```python
from build123d import *

# Parameters (mm, degrees)
SKETCH1_R               = 1.350662837
BOSS_EXTRUDE1_DEPTH     = 3
BOSS_EXTRUDE2_OUTLINE_R = 1.350662837
BOSS_EXTRUDE2_DEPTH     = 5
BOSS_EXTRUDE2_START     = -18.821590418
BOSS_EXTRUDE2_2_DEPTH   = 37.643180836
FILLET1_R               = 0.5
SKETCH5_R               = 2.5
CUT_EXTRUDE1_DEPTH      = 25.78411334
FILLET2_R               = 0.5
FILLET3_R               = 1


with BuildPart() as part:
    # Sketch1 → Boss-Extrude1 (new body)
    with BuildSketch(Plane.XY):
        with BuildLine():
            Line((7.5, 18.821590418), (9.5, 18.821590418))
            Line((9.5, 18.821590418), (9.5, 17.821590418))
            Line((9.5, 17.821590418), (7.5, 15.821590418))
            Line((7.5, 15.821590418), (7.5, 11.821590418))
            ThreePointArc((7.5, 11.821590418), (14, 0), (7.5, -11.821590418))
            Line((7.5, -11.821590418), (7.5, -15.821590418))
            Line((7.5, -15.821590418), (9.5, -17.821590418))
            Line((9.5, -17.821590418), (9.5, -18.821590418))
            Line((9.5, -18.821590418), (7.5, -18.821590418))
            Line((7.5, -18.821590418), (-7.5, -18.821590418))
            Line((-7.5, -18.821590418), (-9.5, -18.821590418))
            Line((-9.5, -18.821590418), (-9.5, -17.821590418))
            Line((-9.5, -17.821590418), (-7.5, -15.821590418))
            Line((-7.5, -15.821590418), (-7.5, -11.821590418))
            ThreePointArc((-7.5, -11.821590418), (-14, 0), (-7.5, 11.821590418))
            Line((-7.5, 11.821590418), (-7.5, 15.821590418))
            Line((-7.5, 15.821590418), (-9.5, 17.821590418))
            Line((-9.5, 17.821590418), (-9.5, 18.821590418))
            Line((-9.5, 18.821590418), (-7.5, 18.821590418))
            Line((-7.5, 18.821590418), (7.5, 18.821590418))
        make_face()
        with Locations((-5, -8.660254038)):
            Circle(SKETCH1_R, mode=Mode.SUBTRACT)
        with Locations((10, 0)):
            Circle(SKETCH1_R, mode=Mode.SUBTRACT)
        with Locations((-5, 8.660254038)):
            Circle(SKETCH1_R, mode=Mode.SUBTRACT)
    extrude(amount=BOSS_EXTRUDE1_DEPTH)

    # Boss-Extrude2: read off the stored shape, not the designer's step
    # Boss-Extrude2 outline → Boss-Extrude2 (add)
    with BuildSketch(Plane(origin=(0, 0, 0), x_dir=(-1, 0, 0), z_dir=(0, 0, -1))):
        with BuildLine():
            Line((-7.5, 15.821590418), (-7.5, 11.821590418))
            ThreePointArc((-7.5, 11.821590418), (-14, 0), (-7.5, -11.821590418))
            Line((-7.5, -11.821590418), (-7.5, -15.821590418))
            Line((-7.5, -15.821590418), (-9.5, -17.821590418))
            Line((-9.5, -17.821590418), (-9.5, -18.821590418))
            Line((-9.5, -18.821590418), (9.5, -18.821590418))
            Line((9.5, -18.821590418), (9.5, -17.821590418))
            Line((9.5, -17.821590418), (7.5, -15.821590418))
            Line((7.5, -15.821590418), (7.5, -11.821590418))
            ThreePointArc((7.5, -11.821590418), (14, 0), (7.5, 11.821590418))
            Line((7.5, 11.821590418), (7.5, 15.821590418))
            Line((7.5, 15.821590418), (9.5, 17.821590418))
            Line((9.5, 17.821590418), (9.5, 18.821590418))
            Line((9.5, 18.821590418), (-9.5, 18.821590418))
            Line((-9.5, 18.821590418), (-9.5, 17.821590418))
            Line((-9.5, 17.821590418), (-7.5, 15.821590418))
        make_face()
        with Locations((5, -8.660254038)):
            Circle(BOSS_EXTRUDE2_OUTLINE_R, mode=Mode.SUBTRACT)
        with Locations((-10, 0)):
            Circle(BOSS_EXTRUDE2_OUTLINE_R, mode=Mode.SUBTRACT)
        with Locations((5, 8.660254038)):
            Circle(BOSS_EXTRUDE2_OUTLINE_R, mode=Mode.SUBTRACT)
    extrude(amount=BOSS_EXTRUDE2_DEPTH)

    # Boss-Extrude2 2 outline → Boss-Extrude2 2 (cut)
    with BuildSketch(Plane(origin=(0, 0, 0), x_dir=(1, 0, 0), z_dir=(0, 1, 0)).offset(BOSS_EXTRUDE2_START)):
        with BuildLine():
            Line((10, 5), (-10, 5))
            ThreePointArc((-10, 5), (0, 0), (10, 5))
        make_face()
    extrude(amount=BOSS_EXTRUDE2_2_DEPTH, mode=Mode.SUBTRACT)

    # Fillet1
    fillet1_edges = [part.edges().sort_by_distance(p)[0] for p in [
        (9.5, 18.321590418, -4.375961595),
        (9.5, -18.321590418, -4.375961595),
        (-9.5, -18.321590418, -4.375961595),
        (-9.5, 18.321590418, -4.375961595),
    ]]
    fillet(fillet1_edges, radius=FILLET1_R)

    # Sketch5 → Cut-Extrude1 (cut, through all)
    with BuildSketch(Plane.XY.offset(3)):
        with Locations((-5, -8.660254038)):
            Circle(SKETCH5_R)
        with Locations((-5, 8.660254038)):
            Circle(SKETCH5_R)
        with BuildLine():
            Line((10, -2.5), (13.774977314, -2.5))
            ThreePointArc((13.774977314, -2.5), (14, 0), (13.774977314, 2.5))
            Line((13.774977314, 2.5), (10, 2.5))
            ThreePointArc((10, 2.5), (7.5, 0), (10, -2.5))
        make_face()
    extrude(amount=-CUT_EXTRUDE1_DEPTH, mode=Mode.SUBTRACT)

    # Fillet2
    fillet2_edges = [part.edges().sort_by_distance(p)[0] for p in [
        (-10, 0, -5),
        (10, -6.148979486, -5),
        (10, 6.148979486, -5),
    ]]
    fillet(fillet2_edges, radius=FILLET2_R)

    # Fillet3
    fillet3_edges = [part.edges().sort_by_distance(p)[0] for p in [
        (13.774977314, 2.5, -2.5),
        (13.774977314, -2.5, -2.5),
    ]]
    fillet(fillet3_edges, radius=FILLET3_R)


solid = part.part
```
CAD build for the part. Positions are in the model's coordinates, mm. A direction names the side the tool comes from. Round coordinates to 2 decimals unless told otherwise and drop trailing zeros. Order: outer loops, then holes, each group sorted by start corner. A loop starts at its lowest first (then second) coordinate and runs counter-clockwise, first axis right, second up. Notation, with made-up numbers: (-17.75, 65) -> (17.25, 65) arc R12 cw to (17.25, 73) -> close; hole circle Ø11 at (57.5, -22.75). An arc over 180 degrees is marked (long way). Write item = value, one per line.
(1) Cut at C-C (x = -7). Write the cut outline in (y, z).
Answers follow:
outline = (-18.82, -2.14) -> (-10.16, -2.14) -> (-10.16, 3) -> (-18.82, 3) -> close; (-7.16, -2.14) -> (7.16, -2.14) -> (7.16, 3) -> (-7.16, 3) -> close; (10.16, -2.14) -> (18.82, -2.14) -> (18.82, 3) -> (10.16, 3) -> close
(2) Cut at A-A (y = 7). Write the cut outline in (x, z).
Answers follow:
outline = (-12.12, -5) -> (-10.25, -5) arc R0.5 ccw to (-9.85, -4.81) arc R12.5 cw to (-6.87, -2.06) -> (-6.87, 3) -> (-12.12, 3) -> close; (-3.13, -0.4) arc R12.5 cw to (9.85, -4.81) arc R0.5 ccw to (10.25, -5) -> (12.12, -5) -> (12.12, 3) -> (-3.13, 3) -> close
(3) Drill centre lines: L1, parallel to Y at x = -5, z = 1; L2, parallel to X at y = -12, z = 1; L3, parallel to X at y = -5, z = -1.25. Where is each one in solid material? Low to high.
Answers follow:
L1 = -18.82 to -11.16, -6.16 to 6.16, 11.16 to 18.82
L2 = -7.5 to 7.5
L3 = -13.08 to -5.45, 5.45 to 13.08
(4) Pull direction Y, two halves, no side cores. Call faces 5 (the flat face through (9.5, -18, 0)), 6 (the flat face through (-0.1, 18.822, 0.5)), 7 (the flat face through (-7.5, 14, 0)): +Y half, -Y half, draft (parallel to the pull), parting line (faces both ways), or undercut.
Answers follow:
face_5 = draft
face_6 = +Y half
face_7 = undercut
(5) 3-axis set-ups, long thin cutter, end or side, ignore diameter. For faces 1 (the cylindrical face through (11.2, 8.4, -0.9)), 2 (the flat face through (9.5, 18, 0)), 3 (the cylindrical face through (-9.063, 18.091, -3.615)), 4 (the cylindrical face through (-9.063, -18.117, -3.615)): which of +Z, -Z, +X, -X, +Y, -Y reach the whole face in a straight line?
Answers follow:
face_1 = +Z, -Z, +X
face_2 = +Z, -Z, +X, +Y
face_3 = -Z, +Y
face_4 = -Z, -Y
(6) Flat gauge pins, fed straight in: P1, Ø12, axis at x = -4, y = -7, coming from the -Z side; P2, Ø0.8, axis at x = 11.5, z = -2.5, coming from the -Y side; P3, Ø1, axis at y = -6.5, z = 2, coming from the +X side; P4, Ø4.5, axis at x = -5, y = -8.66, coming from the -Z side. Where does each tip first touch, or does it go through?
Answers follow:
P1 = -4.93
P2 = -8.53
P3 = 12.65
P4 = through
(7) Cut at D-D (y = 0). Write the cut outline in (x, z).
Answers follow:
outline = (-14, -5) -> (-10.25, -5) arc R0.5 ccw to (-9.85, -4.81) arc R12.5 cw to (7.5, -2.5) -> (7.5, 3) -> (-14, 3) -> close
